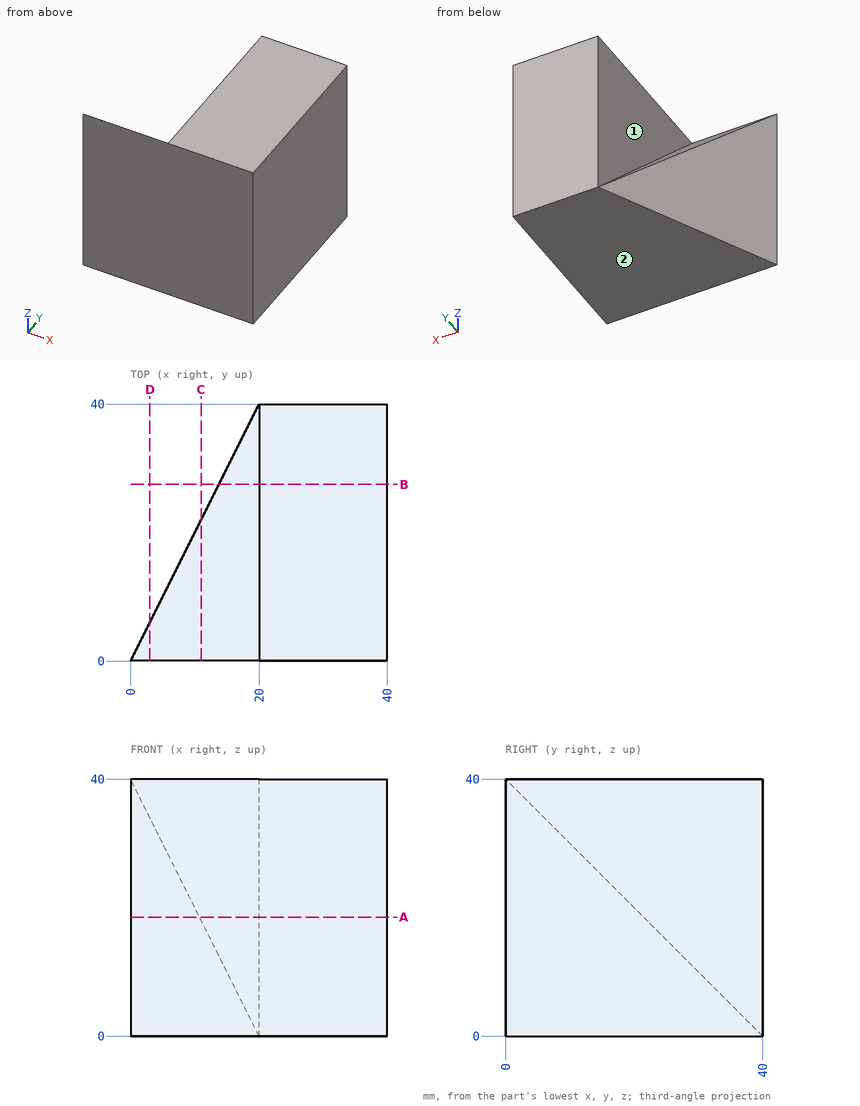
The drawing under review shows one solid part. Ordinate dimensions are in mm from its lowest x, y, z. A direction names the side the tool comes from. Coordinates: 2 decimals unless noted, no trailing zeros. Write each loop counter-clockwise with the first axis right and the second up, starting at its lowest first coordinate (ties: lowest second). Pieces come first, ordered by that corner, then holes. Notation, with made-up numbers: M 69.5,13 L 108.5,13 A8 ccw 108.5,25 Z; hole C 10.5,63 d2. An arc over 180 degrees is marked long. Answer as a JSON object with one key per item and string values.
Item 1: Add section B-B, the plane y = 27.5. Give the boundary of the cut face in (x, z), and give its area (3 significant figures).
Outcome:
{"outline": "M 13.75,0 L 40,0 L 40,40 L 20,40 L 20,12.5 L 13.75,12.5 Z", "area": "878 mm²"}
Item 2: Add section D-D, the plane x = 3. Give the boundary of the cut face in (y, z).
Outcome:
{"outline": "M 0,0 L 6,0 L 6,34 L 0,40 Z"}
Item 3: Add section A-A, the plane z = 18.5. Give the boundary of the cut face in (x, y).
Outcome:
{"outline": "M 0,0 L 40,0 L 40,40 L 20,40 L 20,21.5 L 10.75,21.5 Z"}
Item 4: Wall thickness on probe 1 along X at (y, z) = (16, 37); probe 2 along Z at (x, y) = (11, 4); probe 3 along X at (y, z) = (2, 30): over which ranges is each line inside the solid? List them lowest first.
Outcome:
{"probe 1": "20 to 40", "probe 2": "0 to 36", "probe 3": "1 to 40"}
Item 5: Insertion check: pin 1 Ø6 at (y, z) = (27.5, 16.5) entering from -X; pin 2 Ø3 at (x, y) = (17, 8.5) entering from +Z; pin 3 Ø12 at (x, y) = (31.5, 24) entering from -Z; pin 4 Ø12 at (y, z) = (10.5, 18.5) entering from -X. Each pin has a flat end and moves straight along its axis. Give the tip position at first contact, or say it passes through.
Outcome:
{"pin 1": "x = 12.4", "pin 2": "z = 33", "pin 3": "z = 0", "pin 4": "x = 2.25"}
Item 6: Add section C-C, the plane x = 11. Give the boundary of the cut face in (y, z).
Outcome:
{"outline": "M 0,0 L 22,0 L 22,18 L 0,40 Z"}
Item 7: Machinability: for the marked faces 1 and 2, which of the approach directions +Z, -Z, +X, -X, +Y, -Y give a long, thin tool a straight path to every point of the face, cutting with its end or side? Answer none if there is none.
Outcome:
{"face 1": "+Z, -X, +Y", "face 2": "-Z, +X, -X, +Y, -Y"}
